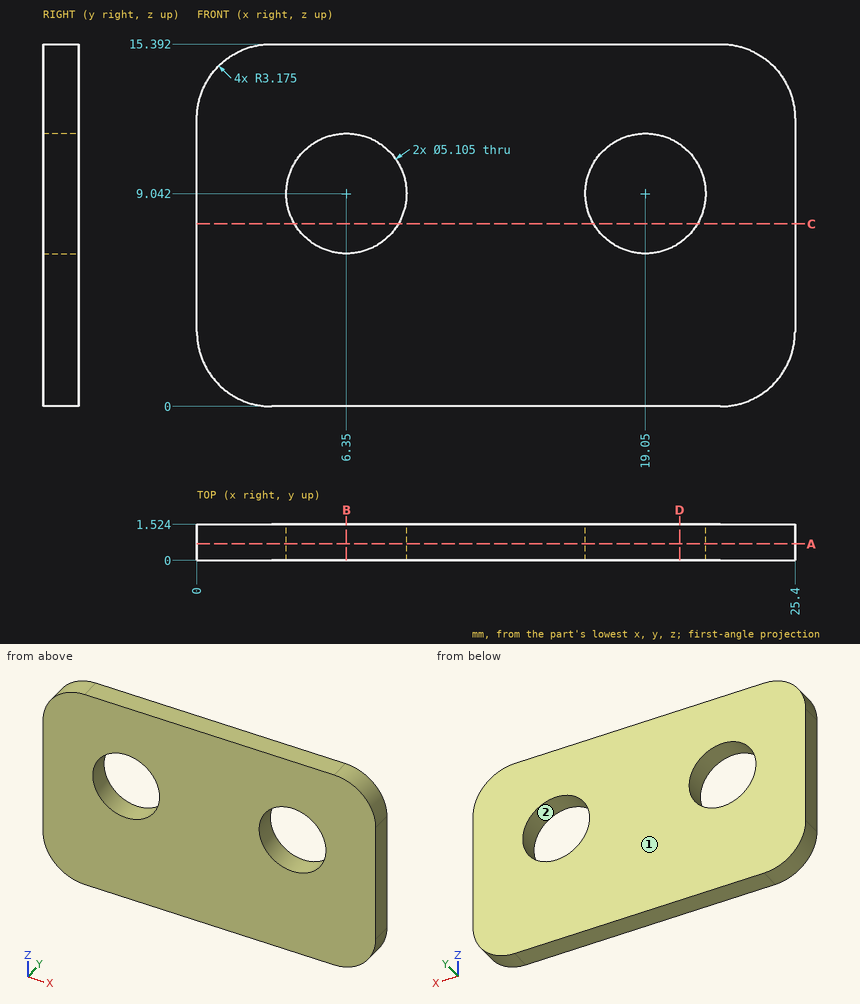
Here's the drawing with two shaded views (mm, measured from the low corner). I have some questions. Give positions to 0.01 mm unless a question says otherwise; leave off trailing zeros. Write each loop counter-clockwise with the first axis right and the second up, starting at its lowest first coordinate (ties: lowest second). Pieces come first, ordered by that corner, then holes. Notation, with made-up numbers: (-2, 34.5) -> (43, 34.5) arc R15 cw to (43, 51.5) -> close; hole circle Ø4 at (-9.5, -31). An arc over 180 degrees is marked (long way). Use one line per item in the form item = value. Start each with the question number.
1. Imagine slicing it at C-C on z = 7.75. List the corners of the cut face in (x, y) for me, plus the area to 3 significant figures.
2. Will this pin go through, and if not, where does the flat tip stop? pin 1 Ø4.5 at (x, z) = (19.05, 9.04) entering from +Y.
3. If I drill on L1, parallel to X at y = 0.4, z = 9; L2, parallel to Z at x = 6.35, y = 0.9 (1 decimal); L3, parallel to Z at x = 8.5, y = 0.35 (1 decimal), over which ranges is the centre line in solid material (lowest first)?
4. Thinking about a two-plate mould opening in X: for the marked faces 1 and 2, which applies, +X half, -X half, draft (parallel to the pull), parting line (faces both ways), or undercut?
5. Imagine slicing it at B-B on x = 6.35. List the corners of the cut face in (y, z) for me (1 decimal).
6. Imagine slicing it at A-A on y = 0.7. State how many separate pieces and enclosed holes the cut face has, plus the area to 3 significant figures.
7. Imagine slicing it at D-D on x = 20.5. List the corners of the cut face in (y, z) for me.
Entries:
q1.outline = (0, 0) -> (4.15, 0) -> (4.15, 1.52) -> (0, 1.52) -> close; (8.55, 0) -> (16.85, 0) -> (16.85, 1.52) -> (8.55, 1.52) -> close; (21.25, 0) -> (25.4, 0) -> (25.4, 1.52) -> (21.25, 1.52) -> close
q1.area = 25.3 mm²
q2.pin_1 = through
q3.L1 = 0 to 3.8, 8.9 to 16.5, 21.6 to 25.4
q3.L2 = 0 to 6.5, 11.6 to 15.4
q3.L3 = 0 to 7.7, 10.4 to 15.4
q4.face_1 = draft
q4.face_2 = undercut
q5.outline = (0, 0) -> (1.5, 0) -> (1.5, 6.5) -> (0, 6.5) -> close; (0, 11.6) -> (1.5, 11.6) -> (1.5, 15.4) -> (0, 15.4) -> close
q6.separate_pieces = 1
q6.enclosed_holes = 2
q6.area = 341 mm²
q7.outline = (0, 0) -> (1.52, 0) -> (1.52, 6.94) -> (0, 6.94) -> close; (0, 11.14) -> (1.52, 11.14) -> (1.52, 15.39) -> (0, 15.39) -> close
